Autodesk Inventor part; units mm, degrees
ref_plane "YZ Plane" through (0, 0, 0) normal (1, 0, 0) x (0, 1, 0)
ref_plane "XZ Plane" through (0, 0, 0) normal (0, 1, 0) x (-1, 0, 0)
ref_plane "XY Plane" through (0, 0, 0) normal (0, 0, 1) x (1, 0, 0)
sketch "Sketch1" plane through (0, 0, 0) normal (0, 0, 1) x (1, 0, 0)
  line L0 (0, 0) -> (50.8, 0)
  line L1 (50.8, 0) -> (50.8, -31.75)
  line L2 (50.8, -31.75) -> (0, -31.75)
  line L3 (0, -31.75) -> (0, 0)
  line L4 (2.8575, 0) -> (8.5725, 0)
  line L5 (8.5725, 0) -> (8.5725, 20.955)
  line L6 (8.5725, 20.955) -> (2.8575, 20.955)
  line L7 (2.8575, 20.955) -> (2.8575, 0)
  line L8 (42.2275, 0) -> (47.9425, 0)
  line L9 (47.9425, 0) -> (47.9425, 20.955)
  line L10 (47.9425, 20.955) -> (42.2275, 20.955)
  line L11 (42.2275, 20.955) -> (42.2275, 0)
  dimension "d1" = 31.75
  dimension "d4" = 5.715
  dimension "d5" = 5.715
  dimension "d21" = 20.955
  dimension "d32" = 50.8
  dimension "d35" = 2.8575
  dimension "d37" = 2.8575
  dimension "d38" = 33.655
extrude "Extrusion1" add sketch "Sketch1" against normal blind 15.875
sketch "Sketch2" plane through (0, 0, 0) normal (0, 0, 1) x (1, 0, 0)
  circle A0 centre (25.4, -15.875) radius 9.5885
  line L0 (50.8, -31.75) -> (0, -31.75)
  line L1 (0, 0) -> (0, -31.75)
  dimension "d10" = 19.177
  dimension "d24" = 15.875
  dimension "d31" = 25.4
extrude "Extrusion2" cut sketch "Sketch2" against normal through all
sketch "Sketch3" plane through (47.9425, 0, 0) normal (1, 0, 0) x (0, 0, -1)
  line L0 (0, 20.955) -> (15.875, 20.955)
  circle A0 centre (7.9375, 13.335) radius 4.7625
  dimension "d13" = 9.525
  dimension "d15" = 7.62
extrude "Extrusion3" cut sketch "Sketch3" against normal up to next
fillet "Fillet2" radius 6.35 2 edges at (50.8, -31.75, -7.9375) (0, -31.75, -7.9375)
fillet "Fillet4" radius 1.5875 8 edges at (50.8, 0, -7.9375) (47.9425, 0, -7.9375) (47.9425, 20.955, -7.9375) (42.2275, 20.955, -7.9375) (8.5725, 20.955, -7.9375) (2.8575, 20.955, -7.9375) (0, 0, -7.9375) (2.8575, 0, -7.9375)
fillet "Fillet5" radius 3.175 2 edges at (8.5725, 0, -7.9375) (42.2275, 0, -7.9375)
sketch "Sketch4" plane through (8.5725, 19.3675, 0) normal (1, 0, 0) x (0, 0, -1)
  circle A0 centre (7.9375, -6.0325) radius 4.7625
  circle A1 centre (7.9375, -6.0325) radius 4.7625
  point P0 (0, -19.3675)
  dimension "d26" = 9.525
extrude "Extrusion4" cut sketch "Sketch4" against normal through all
properties part number "Needle Bearing Mount v2"
The listing builds one solid part. Answer for the finished solid, in the listing's coordinates (mm). A direction names the side the tool comes from. Give positions to 0.01 mm unless a question says otherwise; leave off trailing zeros. Write each loop counter-clockwise with the first axis right and the second up, starting at its lowest first coordinate (ties: lowest second). Pieces come first, ordered by that corner, then holes. Notation, with made-up numbers: (62.25, 69.5) -> (76.25, 69.5) arc R20 ccw to (76.25, 87.5) -> close; hole circle Ø8 at (15.5, 13). An arc over 180 degrees is marked (long way). One line per question, with ' | ' between items. Start each with the question number.
1. Given pin 1 Ø5 at (y, z) = (10.5, -10) entering from +X; pin 2 Ø5 at (x, z) = (19.5, -11.5) entering from +Y; pin 3 Ø8 at (y, z) = (8, -10) entering from -X, each flat-ended and moving along its own axis, determine where each tip first touches the part or whether it passes through.
2. For faces 1 (the flat face through (50.8, -13, -8)), 2 (the flat face through (47.942, 8, -8)), 3 (the flat face through (2.858, 8.6, -6.1)), 4 (the cylindrical face through (42.7, 20.5, -8)), determine the directions among +Z, -Z, +X, -X, +Y, -Y from which every point of the face is accessible in a straight line to the end or side of a thin tool.
3. Section D-D (z = -8) is taken. State how many separate pieces and enclosed holes the cut face has, plus the area to 3 significant figures.
4. For a pull along X with two mould halves and no side action, classify faces 5 (the flat face through (45, 20.955, -8)), 6 (the cylindrical face through (8.1, 20.5, -8)), 7 (the cylindrical face through (50.38, -0.51, -8.05)) as pulls with the +X half, pulls with the -X half, needs draft (parallel to the pull), parting line crosses it, or undercut.
5. Section B-B (y = -14) is taken. Determine the outline of the cut face in (x, z) (3 decimals).
6. Section C-C (y = 14) is taken. Determine the outline of the cut face in (x, z) (1 decimal), plus the area to 3 significant figures.
7. Find the intervals of material crossed by probe 1 along X at (y, z) = (-16, -4); probe 2 along Y at (x, z) = (25.4, -9.75); probe 3 along X at (y, z) = (9.5, -2.25), in increasing order.
Response values:
1) pin 1: x = 47.94 | pin 2: y = 0 | pin 3: x = 2.86
2) face 1: +Z, -Z, +X, +Y, -Y | face 2: +Z, -Z, +X, +Y | face 3: +Z, -Z, -X, +Y | face 4: +Z, -Z, +Y
3) separate pieces: 3 | enclosed holes: 1 | area: 1,440 mm2
4) face 5: needs draft | face 6: undercut | face 7: pulls with the +X half
5) outline: (0, -15.875) -> (15.997, -15.875) -> (15.997, 0) -> (0, 0) -> close; (34.803, -15.875) -> (50.8, -15.875) -> (50.8, 0) -> (34.803, 0) -> close
6) outline: (2.9, -15.9) -> (8.6, -15.9) -> (8.6, -12.7) -> (2.9, -12.7) -> close; (2.9, -3.2) -> (8.6, -3.2) -> (8.6, 0) -> (2.9, 0) -> close; (42.2, -15.9) -> (47.9, -15.9) -> (47.9, -12.7) -> (42.2, -12.7) -> close; (42.2, -3.2) -> (47.9, -3.2) -> (47.9, 0) -> (42.2, 0) -> close | area: 73.6 mm2
7) probe 1: 0 to 15.81, 34.99 to 50.8 | probe 2: -31.75 to -25.46, -6.29 to 0 | probe 3: 2.86 to 8.57, 42.23 to 47.94
